Autodesk Inventor part; units mm, degrees
ref_plane "YZ Plane" through (0, 0, 0) normal (1, 0, 0) x (0, 1, 0)
ref_plane "XZ Plane" through (0, 0, 0) normal (0, 1, 0) x (-1, 0, 0)
ref_plane "XY Plane" through (0, 0, 0) normal (0, 0, 1) x (1, 0, 0)
sketch "Sketch6" plane through (0, 0, 0) normal (0, 1, 0) x (-1, 0, 0)
  line L0 (0, 0) -> (43.9941, -25.4)
  line L1 (43.9941, -25.4) -> (43.9941, -158.75)
  line L2 (43.9941, -158.75) -> (44.6063, -159.1035)
  line L3 (43.9941, -158.75) -> (44.701, -158.75) construction
  line L4 (43.0188, -161.8531) -> (40.8191, -160.5831)
  line L5 (40.8191, -160.5831) -> (40.8191, -27.2331)
  line L6 (40.8191, -27.2331) -> (-1.5875, -2.7496)
  line L7 (-1.5875, -2.7496) -> (0, 0)
  line L8 (0, 0) -> (22.7499, 0) construction
  line L9 (43.0188, -161.8531) -> (44.6063, -159.1035)
  dimension "d15" = 50.8
  dimension "d17" = 133.35
  dimension "d21" = 3.175
  dimension "d22" = 30
  dimension "d27" = 120
  dimension "d29" = 2.54
  dimension "d30" = 90
extrude "Extrusion5" add sketch "Sketch6" along normal blind 152.4
properties part number "flap"
CAD build for the part. Positions are in the model's coordinates, mm. A direction names the side the tool comes from. Round coordinates to 2 decimals unless told otherwise and drop trailing zeros. Write each loop counter-clockwise with the first axis right and the second up, starting at its lowest first coordinate (ties: lowest second). Pieces come first, ordered by that corner, then holes. Notation, with made-up numbers: (24, 53.25) -> (35, 53.25) arc R26 cw to (35, 86.25) -> close; hole circle Ø10 at (85.5, -15.75). An arc over 180 degrees is marked (long way). Answer in a Markdown table with one row per item. Add a question column.
Item 1: Saw through at B-B, the plane z = -81.5. Write the cut outline in (x, y).
Item 2: Saw through at C-C, the plane x = -10.5. Write the cut outline in (y, z), then the cut area to 3 significant figures.
Item 3: Drill centre lines: line 1 (X direction, y = 95.5, z = -91); line 2 (Z direction, x = -21.5, y = 116); line 3 (Z direction, x = -7, y = 53). Where is each one in solid material? Low to high. Write a range as from..to.
Item 4: Saw through at A-A, the plane y = 22. Write the cut outline in (x, z), then the cut area to 3 significant figures.
Item 5: Drop flat-ended pins along their axis: pin 1 Ø4 at (y, z) = (40, -86.5) entering from +X; pin 2 Ø10 at (x, y) = (-24, 81.5) entering from +Z; pin 3 Ø6 at (x, y) = (-33.5, 96.5) entering from -Z. Give the stop position or say it passes through.
Item 6: Which spindle directions (+Z, -Z, +X, -X, +Y, -Y) get a long thin tool onto all of the face, cutting with end or side? Do faces 1 (the face through (-43.994, 75, -91)), 2 (the face through (-42, 152.4, -69)), 3 (the face through (-40.819, 75, -95)). Say none if no direction does.
Findings below:
| question | item | result |
|---|---|---|
| 1 | outline | (-43.99, 0) -> (-40.82, 0) -> (-40.82, 152.4) -> (-43.99, 152.4) -> close |
| 2 | outline | (0, -9.73) -> (152.4, -9.73) -> (152.4, -6.06) -> (0, -6.06) -> close |
| 2 | area | 559 mm^2 |
| 3 | line 1 | x = -43.99..-40.82 |
| 3 | line 2 | z = -16.08..-12.41 |
| 3 | line 3 | z = -7.71..-4.04 |
| 4 | outline | (-44.61, -159.1) -> (-43.02, -161.85) -> (-40.82, -160.58) -> (-40.82, -27.23) -> (1.59, -2.75) -> (0, 0) -> (-43.99, -25.4) -> (-43.99, -158.75) -> close |
| 4 | area | 587 mm^2 |
| 5 | pin 1 | stops at x = -40.82 |
| 5 | pin 2 | stops at z = -10.97 |
| 5 | pin 3 | stops at z = -24.74 |
| 6 | face 1 | +Z, -X, +Y, -Y |
| 6 | face 2 | +Z, -Z, +X, -X, +Y |
| 6 | face 3 | -Z, +X, +Y, -Y |
